Answer from the drawing. Dimensions are ordinates in mm from the lowest x, y and z of the part. Give positions to 0.01 mm unless a question says otherwise; leave off trailing zeros. Order: outer loops, then holes, each group sorted by start corner. A loop starts at its lowest first (then second) coordinate and runs counter-clockwise, first axis right, second up. Notation, with made-up numbers: (52, 30.5) - (90, 30.5) arc R35 ccw to (90, 67.5) - close; hole circle Ø5 at (67, 68.5). An arc over 180 degrees is marked (long way). Use a Markdown table: item, result. Add a question column.
1) Find section B-B, the plane x = 6.25. Determine the outline of the cut face in (y, z).
2) Find section C-C, the plane y = 0.3. Determine the outline of the cut face in (x, z).
3) Straight lines are drawn through the part: line 1 (X direction, y = 0.35, z = 6.25); line 2 (X direction, y = 0.35, z = 7.25); line 3 (Z direction, x = 7.75, y = 0.3). For each, find the intervals that lie inside material, in ascending order.
4) Find section A-A, the plane z = 10. Determine the outline of the cut face in (x, y), plus the area to 3 significant figures.
5) Find section D-D, the plane x = 2.5. Determine the outline of the cut face in (y, z).
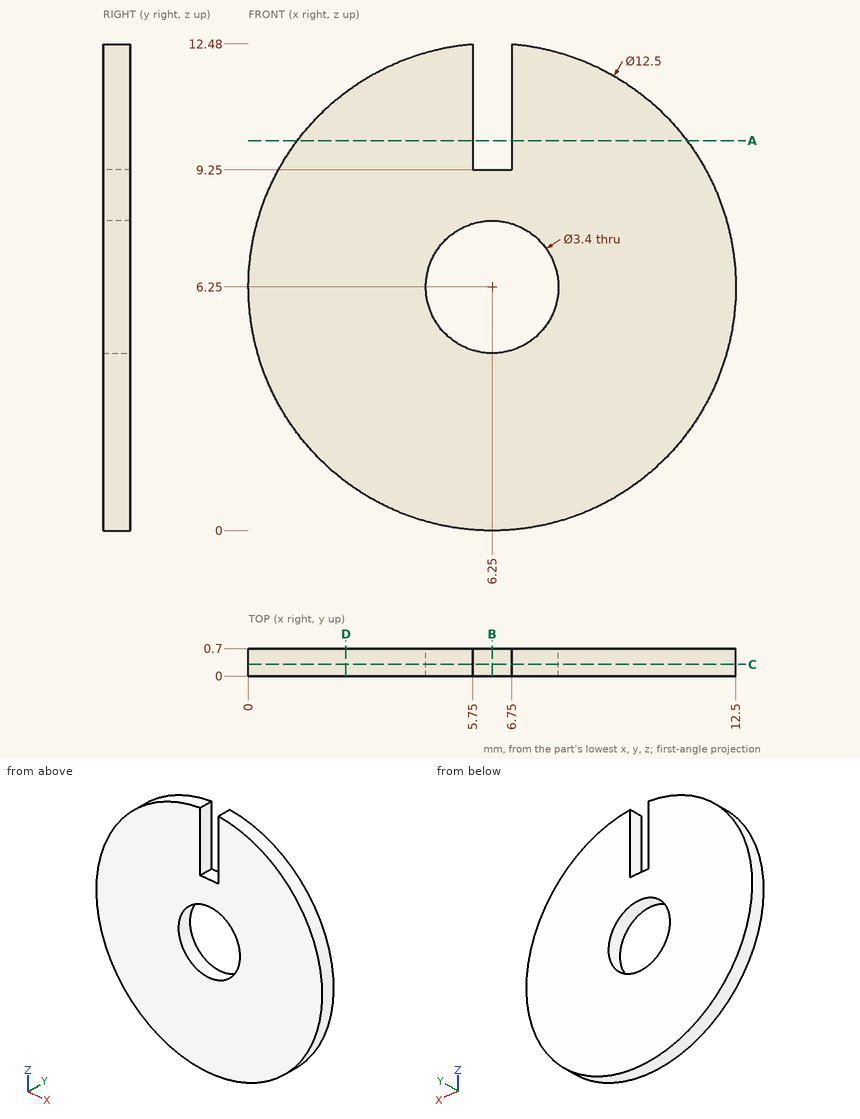
The answers:
| question | item | result |
|---|---|---|
| 1 | outline | (0, 0) - (0.7, 0) - (0.7, 4.55) - (0, 4.55) - close; (0, 7.95) - (0.7, 7.95) - (0.7, 9.25) - (0, 9.25) - close |
| 2 | outline | (5.75, 9.25) - (5.75, 12.48) arc R6.25 ccw (long way) to (6.75, 12.48) - (6.75, 9.25) - close; hole circle Ø3.4 at (6.25, 6.25) |
| 3 | line 1 | 0 to 4.55, 7.95 to 12.5 |
| 3 | line 2 | 0.08 to 4.88, 7.62 to 12.42 |
| 3 | line 3 | 0.18 to 5.45, 7.05 to 12.32 |
| 4 | outline | (1.25, 0) - (5.75, 0) - (5.75, 0.7) - (1.25, 0.7) - close; (6.75, 0) - (11.25, 0) - (11.25, 0.7) - (6.75, 0.7) - close |
| 4 | area | 6.30 mm2 |
| 5 | outline | (0, 1.25) - (0.7, 1.25) - (0.7, 11.25) - (0, 11.25) - close |
